```python
from build123d import *

# Parameters (mm, degrees)
BOSS_EXTRUDE1_DEPTH = 25.4
SKETCH2_R           = 25.4
BOSS_EXTRUDE2_DEPTH = 304.8


with BuildPart() as part:
    # Sketch1 → Boss-Extrude1 (new body)
    with BuildSketch(Plane.XY):
        with BuildLine():
            add(Edge.make_bspline(
                [(471.400045341, 247.723418726), (471.253377656, 237.207919779), (470.967830054, 216.735274463), (467.254101988, 187.082974518), (461.8496739, 159.345276671), (453.870836324, 133.784385037), (444.180642621, 110.205863151), (432.473184544, 88.68343609), (419.069697548, 69.152650509), (403.779500623, 51.811813407), (386.883763515, 36.465486204), (368.07226234, 23.500783632), (347.87819623, 12.143124499), (326.005689501, 3.075456628), (302.798046482, -3.945259965), (278.356817124, -8.845510147), (252.854402734, -12.087794668), (235.433814702, -12.457415416), (226.578825663, -12.645295851)],
                knots=[0, 0, 0, 0, 1.243239104, 2.420464626, 3.5298884, 4.582278609, 5.582746481, 6.541150455, 7.475403342, 8.379003492, 9.270392267, 10.168465759, 11.076013954, 12.006683471, 12.963517291, 13.939882109, 14.95282976, 16, 16, 16, 16], degree=3))
            add(Edge.make_bspline(
                [(226.578825663, -12.645295851), (218.352164012, -12.538505316), (201.941331975, -12.325475825), (177.573248938, -10.221700143), (153.862654705, -6.662758999), (130.879483257, -3.263565991), (109.182795007, 1.737149247), (88.715264824, 6.718897763), (69.935399564, 12.530624018), (58.098073578, 16.817649327), (52.446882793, 18.864293811)],
                knots=[0, 0, 0, 0, 1.110164411, 2.214594747, 3.297432602, 4.346158016, 5.348621489, 6.300893974, 7.188839411, 8, 8, 8, 8], degree=3))
            Line((52.446882793, 18.864293811), (52.446882793, 139.305554296))
            add(Edge.make_bspline(
                [(52.446882793, 139.305554296), (64.874628492, 133.075868175), (90.412266994, 120.274554406), (125.374016113, 109.704702571), (155.301093725, 103.008826714), (179.811466542, 99.962362648), (205.657832859, 97.41723642), (223.461985851, 97.289275944), (232.590523691, 97.223668102)],
                knots=[0, 0, 0, 0, 1.33626015, 2.745866344, 3.501339399, 4.286907587, 5.121663978, 6, 6, 6, 6], degree=3))
            add(Edge.make_bspline(
                [(232.590523691, 97.223668102), (239.158269417, 97.352295207), (251.76305327, 97.599155684), (269.927956029, 99.212302505), (286.582747303, 102.077475814), (301.811701074, 106.180132756), (315.556993667, 111.584001003), (327.916187793, 118.068049642), (339.074197486, 125.536988417), (348.820608618, 134.331311428), (357.487925057, 144.147017107), (364.581237124, 155.14551392), (370.818795453, 166.942817171), (377.159465823, 184.562779609), (382.483224001, 209.282497228), (383.152996334, 229.862905592), (383.504874178, 240.675221038)],
                knots=[0, 0, 0, 0, 1.150469122, 2.207974428, 3.191023612, 4.107189959, 4.965818341, 5.772540898, 6.548058224, 7.311004937, 8.065940222, 8.834721628, 9.59805231, 10.398484715, 12.107874311, 14, 14, 14, 14], degree=3))
            add(Edge.make_bspline(
                [(383.504874178, 240.675221038), (383.375775152, 246.629845256), (383.125140139, 258.190252509), (380.338077986, 274.806688854), (376.07447805, 290.096343088), (367.854208023, 308.522003494), (354.046911722, 329.449339694), (333.034344764, 351.517108283), (308.623384124, 371.497142004), (280.873457154, 389.02389929), (251.61970563, 406.27894442), (221.506803957, 423.847060642), (191.575771198, 442.899613424), (161.963381352, 463.038143438), (134.213750684, 486.282103081), (113.808817585, 508.88596626), (99.373288206, 528.958664647), (89.850872373, 545.572294954), (81.174232028, 563.263750696), (73.576338245, 582.335707349), (67.531929478, 603.000329232), (63.295829594, 625.423786322), (60.478492711, 649.675796329), (60.240534913, 666.460677888), (60.116980277, 675.175878486)],
                knots=[0, 0, 0, 0, 0.683481112, 1.326921685, 1.929962516, 2.50227757, 3.638507422, 4.789972352, 5.991472863, 7.25317922, 8.556146245, 9.89452332, 11.257815158, 12.632065813, 14.006385259, 15.406082955, 16.117620294, 16.843365227, 17.603177928, 18.380093015, 19.199067628, 20.072523982, 20.999198172, 22, 22, 22, 22], degree=3))
            add(Edge.make_bspline(
                [(60.116980277, 675.175878486), (60.266347944, 682.992198254), (60.563202146, 698.526399296), (63.268407253, 721.702673865), (67.029218595, 744.756252708), (72.938939866, 767.448084012), (80.167383133, 789.646297398), (89.804124706, 810.536229263), (101.036631814, 830.225911242), (114.138002232, 848.513903833), (129.090687529, 865.465550925), (146.225980036, 880.584019249), (165.180405766, 894.200695058), (186.25374332, 905.817065987), (209.267887705, 915.423849913), (234.463660866, 922.322523346), (261.770601719, 926.159928277), (280.672245102, 926.743908945), (290.427204715, 927.045295851)],
                knots=[0, 0, 0, 0, 0.975284822, 1.938286936, 2.909635212, 3.888688786, 4.862446742, 5.819714805, 6.754769447, 7.688271271, 8.623047391, 9.570000944, 10.534585516, 11.530702109, 12.567083431, 13.640560543, 14.782315582, 16, 16, 16, 16], degree=3))
            add(Edge.make_bspline(
                [(290.427204715, 927.045295851), (295.821792555, 926.991722181), (307.119137631, 926.879528209), (324.527852683, 924.980301832), (342.762087373, 922.723310686), (361.204928023, 918.9146153), (379.753810568, 915.252650517), (397.872810434, 910.343585066), (415.259940193, 905.344049371), (426.429567097, 901.521556255), (431.805758331, 899.681704829)],
                knots=[0, 0, 0, 0, 0.894821679, 1.873935432, 2.90385038, 3.942982464, 4.997879381, 6.040990772, 7.057085046, 8, 8, 8, 8], degree=3))
            Line((431.805758331, 899.681704829), (431.805758331, 787.739741555))
            add(Edge.make_bspline(
                [(431.805758331, 787.739741555), (419.733337143, 792.567334637), (395.961042108, 802.073544308), (359.459798072, 811.490129789), (323.753844875, 817.963444445), (300.128004953, 818.8267049), (288.561505328, 819.249331217)],
                knots=[0, 0, 0, 0, 1.056204648, 2.079815483, 3.059935496, 4, 4, 4, 4], degree=3))
            add(Edge.make_bspline(
                [(288.561505328, 819.249331217), (282.752570383, 819.122689661), (271.45602877, 818.87641188), (255.109911254, 817.188203241), (239.881672867, 814.614015324), (225.951841889, 810.623314646), (213.116176925, 805.672302763), (201.514790252, 799.441268731), (191.040837515, 792.170464752), (178.867178614, 781.047066068), (166.220178449, 764.674130027), (155.599605332, 741.712519513), (148.992646474, 715.757338896), (148.348308943, 697.398939659), (148.01215144, 687.821174337)],
                knots=[0, 0, 0, 0, 0.952372428, 1.852063221, 2.692205999, 3.481287024, 4.2240212, 4.943845178, 5.635379706, 6.309142243, 7.641770197, 8.995046942, 10.432285145, 12, 12, 12, 12], degree=3))
            add(Edge.make_bspline(
                [(148.01215144, 687.821174337), (148.140595609, 681.866602086), (148.389959273, 670.306295722), (151.197000805, 653.623427204), (155.491262386, 638.151905383), (163.526964206, 619.363875789), (177.574982405, 598.255795043), (198.321298675, 575.633877137), (223.159092318, 555.954749965), (250.598364534, 537.810758968), (280.141752918, 520.983163901), (309.875051442, 502.801163048), (340.136869423, 484.327686063), (369.344089464, 463.38289759), (397.383997281, 440.065868192), (417.599449013, 416.756221958), (431.84436681, 396.186226446), (441.768261809, 379.422271106), (450.322403238, 361.273846123), (457.904994803, 341.861518304), (464.016933769, 320.870667906), (468.213349889, 298.093157172), (471.031668208, 273.498795578), (471.274503264, 256.507607726), (471.400045341, 247.723418726)],
                knots=[0, 0, 0, 0, 0.67806531, 1.316407357, 1.922242701, 2.504478499, 3.638316715, 4.792219623, 5.99029874, 7.239775474, 8.539190492, 9.864250055, 11.212536268, 12.578556635, 13.958200154, 15.359258983, 16.078046046, 16.808815146, 17.576792489, 18.362220191, 19.182266718, 20.064269398, 20.999256344, 22, 22, 22, 22], degree=3))
        make_face()
    extrude(amount=BOSS_EXTRUDE1_DEPTH)

    # Sketch2 → Boss-Extrude2 (add)
    with BuildSketch(Plane(origin=(0, 0, 0), x_dir=(-1, 0, 0), z_dir=(0, 0, -1))):
        with Locations(Location((-360.220944294, 860.84485697, 0), (0, 0, 180))):
            Circle(SKETCH2_R)
        with Locations(Location((-120.389931068, 47.62475465, 0), (0, 0, 180))):
            Circle(SKETCH2_R)
    extrude(amount=BOSS_EXTRUDE2_DEPTH)


solid = part.part
```
Geometry check sheet. Reference: the model listing, model coordinates, mm. A direction names the side the tool comes from. Coordinates: 2 decimals unless noted, no trailing zeros. Order: outer loops, then holes, each group sorted by start corner. A loop starts at its lowest first (then second) coordinate and runs counter-clockwise, first axis right, second up.
Item 1: Scan lines: line 1 along Z through (x, y) = (395.5, 411); line 2 along Y through (x, z) = (359.5, -256.5); line 3 along X through (y, z) = (879.5, -61.5). Record each from-to range of solid material in increasing order.
Item 2: Tool access check on faces 1 (the cylindrical face through (371.9, 883.4, -150.3)), 2 (the flat face through (265, 464, 25.4)), 3 (the flat face through (431.806, 844, 13)). Record the directions out of +Z, -Z, +X, -X, +Y, -Y that give a thin tool (end or side, any length) a straight path to the whole face; none if there is none.
Item 3: Section check B-B (z = -49.5). Enter the section's corners in (x, y).
Item 4: Depth check by flat-ended pin: pin 1 (10 mm diameter, centred on x = 330, y = 392.5, fed in from -Z); pin 2 (7.5 mm diameter, centred on y = 857, z = 18.5, fed in from +X). Enter the tip coordinate at first touch or a pass-through.
Item 5: Section check A-A (x = 259). Count the separate pieces of the cut face and the enclosed holes in it, plus the area to 3 significant figures.
Check sheet entries:
1. line 1: z = 0 to 25.4
1. line 2: y = 835.46 to 886.23
1. line 3: x = 342.98 to 377.46
2. face 1: -Z
2. face 2: +Z, +X, -X, +Y, -Y
2. face 3: +Z, -Z, +X, +Y
3. outline: circle Ø50.8 at (120.39, 47.62); circle Ø50.8 at (360.22, 860.84)
4. pin 1: stops at z = 0
4. pin 2: stops at x = 431.81
5. separate pieces: 3
5. enclosed holes: 0
5. area: 8,850 mm2
